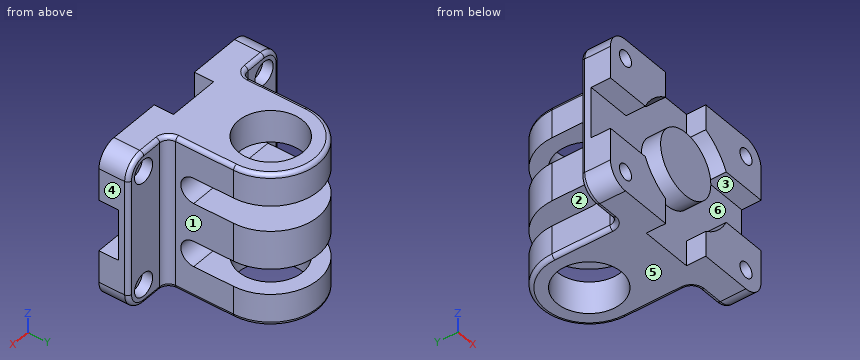
from build123d import *

# Parameters (mm, degrees)
EXTRUDE_1_DEPTH              = 60
SKETCH_3_W                   = 40
SKETCH_3_H                   = 15
CUT_EXTRUDE_1_DEPTH          = 76
CUT_EXTRUDE_1_DEPTH_BACK     = 76
SKETCH_4_R                   = 25
CUT_EXTRUDE_2_DEPTH          = 25
CUT_EXTRUDE_3_REACH          = 77
SKETCH_5_R                   = 7
FILLET_1_R                   = 15
HOLE_WIZARD_M2_1_D           = 12
HOLE_WIZARD_M2_1_CBORE_D     = 18
HOLE_WIZARD_M2_1_CBORE_DEPTH = 8
FILLET_2_R                   = 3
SKETCH_11_R                  = 45
CUT_EXTRUDE_4_DEPTH          = 15
SKETCH_12_R                  = 25
EXTRUDE_2_DEPTH              = 15


with BuildPart() as part:
    # 스케치1 → 보스-돌출1 (new body, symmetric)
    with BuildSketch(Plane.XY):
        with BuildLine():
            Line((-75, 0), (-20, 0))
            Line((-20, 0), (-20, 15))
            Line((-20, 15), (20, 15))
            Line((20, 15), (20, 0))
            Line((20, 0), (75, 0))
            Line((75, 0), (75, 23))
            Line((75, 23), (44, 23))
            ThreePointArc((44, 23), (39.050252532, 25.050252532), (37, 30))
            Line((37, 30), (37, 75))
            ThreePointArc((37, 75), (0, 112), (-37, 75))
            Line((-37, 75), (-37, 30))
            ThreePointArc((-37, 30), (-39.050252532, 25.050252532), (-44, 23))
            Line((-44, 23), (-75, 23))
            Line((-75, 23), (-75, 0))
        make_face()
    extrude(amount=EXTRUDE_1_DEPTH, both=True)

    # 스케치3 → 컷-돌출1 (cut, two sides)
    with BuildSketch(Plane(origin=(0, 0, 0), x_dir=(0, 0, -1), z_dir=(1, 0, 0))) as cut_extrude_1_sk:
        with BuildLine():
            Line((-35, 44), (-35, 156))
            ThreePointArc((-35, 156), (-25, 166), (-15, 156))
            Line((-15, 156), (-15, 44))
            ThreePointArc((-15, 44), (-25, 34), (-35, 44))
        make_face()
        with BuildLine():
            Line((35, 44), (35, 156))
            ThreePointArc((35, 156), (25, 166), (15, 156))
            Line((15, 156), (15, 44))
            ThreePointArc((15, 44), (25, 34), (35, 44))
        make_face()
        with Locations((0, 7.5)):
            Rectangle(SKETCH_3_W, SKETCH_3_H)
    extrude(amount=CUT_EXTRUDE_1_DEPTH, mode=Mode.SUBTRACT)
    extrude(cut_extrude_1_sk.sketch, amount=-CUT_EXTRUDE_1_DEPTH_BACK, mode=Mode.SUBTRACT)

    # 스케치4 → 컷-돌출2 (cut)
    with BuildSketch(Plane.XY.offset(60)):
        with Locations((0, 75)):
            Circle(SKETCH_4_R)
    cut_extrude_2 = extrude(amount=-CUT_EXTRUDE_2_DEPTH, mode=Mode.SUBTRACT)

    # 대칭 복사1: 컷-돌출2 across plane
    add(cut_extrude_2.mirror(Plane.XY), mode=Mode.SUBTRACT)

    # 스케치5 → 컷-돌출3 (cut, up to next)
    with BuildSketch(Plane.XY.offset(15), mode=Mode.PRIVATE) as cut_extrude_3_sk1:
        with Locations((0, 75)):
            Circle(SKETCH_5_R)
    cut_extrude_3_tool1 = extrude(cut_extrude_3_sk1.sketch, amount=-CUT_EXTRUDE_3_REACH, mode=Mode.PRIVATE) & part.part
    add(cut_extrude_3_tool1.solids().sort_by_distance((0, 75, 15))[0], mode=Mode.SUBTRACT)

    # 필렛1
    fillet_1_edges = [part.edges().sort_by_distance(p)[0] for p in [
        (75, 11.5, -60),
        (-75, 11.5, -60),
        (75, 11.5, 60),
        (-75, 11.5, 60),
    ]]
    fillet(fillet_1_edges, radius=FILLET_1_R)

    # M2 소켓 머리 캡 나사용 카운터보어1 (through all)
    with Locations(Plane(origin=(0, 23, 0), x_dir=(1, 0, 0), z_dir=(0, 1, 0))):
        with Locations((-60, 45), (-60, -45)):
            hole_wizard_m2_1 = CounterBoreHole(HOLE_WIZARD_M2_1_D / 2, HOLE_WIZARD_M2_1_CBORE_D / 2, HOLE_WIZARD_M2_1_CBORE_DEPTH)

    # 대칭 복사2: M2 소켓 머리 캡 나사용 카운터보어1 across plane
    add(hole_wizard_m2_1.mirror(Plane(origin=(0, 0, 0), x_dir=(0, 0, 1), z_dir=(1, 0, 0))), mode=Mode.SUBTRACT)

    # 필렛2
    fillet_2_edges = [part.edges().sort_by_distance(p)[0] for p in [
        (-75, 23, 0),
        (-52, 23, -60),
        (52, 23, -60),
        (-70.606601718, 23, 55.606601718),
        (-70.606601718, 23, -55.606601718),
        (-39.050252532, 25.050252532, -60),
        (75, 23, 0),
        (52, 23, 60),
        (70.606601718, 23, 55.606601718),
        (70.606601718, 23, -55.606601718),
        (-37, 52.5, -60),
        (0, 112, -60),
        (37, 52.5, -60),
        (39.050252532, 25.050252532, -60),
        (39.050252532, 25.050252532, 60),
        (37, 52.5, 60),
        (0, 112, 60),
        (-37, 52.5, 60),
        (-39.050252532, 25.050252532, 60),
        (-52, 23, 60),
    ]]
    fillet(fillet_2_edges, radius=FILLET_2_R)

    # 스케치11 → 컷-돌출4 (cut)
    with BuildSketch(Plane.XZ):
        Circle(SKETCH_11_R)
    extrude(amount=-CUT_EXTRUDE_4_DEPTH, mode=Mode.SUBTRACT)

    # 스케치12 → 보스-돌출2 (add)
    with BuildSketch(Plane.XZ.offset(-15)):
        Circle(SKETCH_12_R)
    extrude(amount=EXTRUDE_2_DEPTH)


solid = part.part
The model under review builds one solid part; all positions refer to its coordinate system, in mm. Face numbers are marked on the shaded views. A direction names the side the tool comes from. Coordinates: 2 decimals unless noted, no trailing zeros. Write each loop counter-clockwise with the first axis right and the second up, starting at its lowest first coordinate (ties: lowest second). Pieces come first, ordered by that corner, then holes. Notation, with made-up numbers: M 33,77.5 L 77,77.5 A24 cw 77,107.5 Z; hole C 60.25,-6.75 d6. An arc over 180 degrees is marked long. Put each result on its own line as item: value.
1) Draft analysis for pull direction Z (two halves, no side actions). For the marked faces 4, 5 and 6, state which applies: released by +Z, released by -Z, zero draft, split by the parting line, or undercut.
Computed:
face 4: zero draft
face 5: released by -Z
face 6: undercut
2) Clearance check with flat-ended pins moving along their axes: pin 1 Ø15.5 at (x, z) = (60, 45) entering from +Y; pin 2 Ø14.5 at (x, z) = (-61, 47.5) entering from +Y; pin 3 Ø4 at (x, y) = (17.5, 81) entering from -Z. State where each tip first meets the part, or that it passes through.
Computed:
pin 1: stops at y = 15
pin 2: stops at y = 23
pin 3: stops at z = -15
3) For the marked faces 1, 2 and 3, list the 3-axis set-ups (+Z, -Z, +X, -X, +Y, -Y) from which the entire face can be reached by the end or side of a thin tool; tool diameter is ignored.
Computed:
face 1: +Z, -Z, +X, +Y
face 2: +X, -X, +Y
face 3: +X, -Y
4) Add section D-D on y = 63. Give the boundary of the cut face in (x, z).
Computed:
outline: M -37,-57 A3 ccw -34,-60 L -21.93,-60 L -21.93,-35 L -37,-35 Z; M -37,-15 L 37,-15 L 37,15 L -37,15 Z; M -37,35 L -21.93,35 L -21.93,60 L -34,60 A3 ccw -37,57 Z; M 21.93,-60 L 34,-60 A3 ccw 37,-57 L 37,-35 L 21.93,-35 Z; M 21.93,35 L 37,35 L 37,57 A3 ccw 34,60 L 21.93,60 Z
5) Add section A-A on y = 11. State how many separate pieces and enclosed holes the cut face has, then the cut area to 3 significant figures.
Computed:
separate pieces: 5
enclosed holes: 4
area: 9,110 mm2
6) Add section B-B on z = 0. Give the boundary of the cut face in (x, y).
Computed:
outline: M -75,15 L -25,15 L -25,0 L 25,0 L 25,15 L 75,15 L 75,20 A3 ccw 72,23 L 44,23 A7 cw 37,30 L 37,75 A37 ccw -37,75 L -37,30 A7 cw -44,23 L -72,23 A3 ccw -75,20 Z; hole C 0,75 d14
7) Wall thickness on probe 1 along Z at (x, y) = (-60, 8.25); probe 2 along Z at (x, y) = (-28, 70.5); probe 3 along X at (y, z) = (20, -45): over which ranges is each line inside the solid? List them lowest first. Write a range as [from, to].
Computed:
probe 1: z = [-60, -51], [-39, -20], [20, 39], [51, 60]
probe 2: z = [-60, -35], [-15, 15], [35, 60]
probe 3: x = [-75, -69], [-51, 51], [69, 75]
